Could you check a few things on this model? Use its own coordinates, in mm. A direction names the side the tool comes from. Coordinates: 2 decimals unless noted, no trailing zeros. Write each loop counter-clockwise with the first axis right and the second up, starting at its lowest first coordinate (ties: lowest second). Pieces come first, ordered by that corner, then holes.
Item 1: For P1, Ø3, axis at x = 7, z = 11.5, coming from the +Y side; P2, Ø6.5, axis at y = 8, z = 7.5, coming from the +X side; P3, Ø1, axis at x = 3, z = 10, coming from the +Y side; P4, Ø3, axis at y = -24.5, z = 5.5, coming from the -X side, each with a flat end and sliding along its axis, tell me the tip position at first contact or that it passes through.
Item 2: I want a section at A-A on z = 7.5. Please give me the cut outline in (x, y), then the cut area to 4 significant figures.
Item 3: Thinking about a two-plate mould opening in Z: for faces 4 (the flat face through (10, -13, 15)), 5 (the cylindrical face through (2.46, 6.39, 11.38)), 6 (the flat face through (2.5, 15, 7.5)), which applies, +Z half, -Z half, draft (parallel to the pull), parting line (faces both ways), or undercut?
Item 4: I want a section at B-B on x = 2.25. Please give me the cut outline in (y, z), then the cut area to 3 significant figures.
Item 5: Which directions (+Z, -Z, +X, -X, +Y, -Y) give clear straight access to the entire face, cutting with the end or side of a thin tool? Please do faces 1 (the flat face through (9, 0, 7)), 2 (the flat face through (11, -35, 7)), 3 (the flat face through (4, -5, 7)).
Item 6: I want a section at D-D on x = 10.5. Please give me the cut outline in (y, z).
Item 7: If I drill on probe 1 along Y at (x, z) = (3.15, 7.5); probe 2 along Z at (x, y) = (1.4, 8); probe 3 along X at (y, z) = (-33, 9), over which ranges is the centre line in solid material (lowest first)?
Item 8: I want a section at C-C on y = -20. Please give me the cut outline in (x, z), then the cut area to 3 significant figures.
Solid Edge part; units mm, degrees
sketch "Sketch1" plane through (0, 0, 0) normal (0, -1, 0) x (1, 0, 0)
  line L0 (13.5, 0) -> (0, 0)
  line L1 (0, 0) -> (0, 15)
  line L2 (0, 15) -> (13.5, 15)
  line L3 (13.5, 15) -> (13.5, 0)
extrude "Protrusion1" add sketch "Sketch1" along normal blind 5
sketch "Sketch2" plane through (18.75, -5, 7.5) normal (0, -1, 0) x (1, 0, 0)
  line L0 (-10.25, -7.5) -> (-10.25, 7.5)
  line L1 (-10.25, 7.5) -> (-5.25, 7.5)
  line L2 (-5.25, 7.5) -> (-5.25, -7.5)
  line L3 (-5.25, -7.5) -> (-10.25, -7.5)
extrude "ExtrudedProtrusion_2" add sketch "Sketch2" along normal blind 30
sketch "Sketch3" plane through (18.75, 0, 7.5) normal (0, 1, 0) x (-1, 0, 0)
  line L0 (13.75, -7.5) -> (13.75, 7.5)
  line L1 (13.75, 7.5) -> (18.75, 7.5)
  line L2 (18.75, 7.5) -> (18.75, -7.5)
  line L3 (18.75, -7.5) -> (13.75, -7.5)
extrude "ExtrudedProtrusion_3" add sketch "Sketch3" along normal blind 15
sketch "Sketch4" plane through (13.5, -17.5, 7.5) normal (1, 0, 0) x (0, 1, 0)
  circle A0 centre (-2.5, 0) radius 4
extrude "Cutout1" cut sketch "Sketch4" against normal through all
sketch "Sketch5" plane through (0, 5, 7.5) normal (-1, 0, 0) x (0, -1, 0)
  circle A0 centre (-3, 0) radius 4
extrude "Cutout2" cut sketch "Sketch5" against normal through all
fillet "Round1" radius 7 2 edges at (2.5, 15, 15) (2.5, 15, 0)
hole "Hole_1" at (0, 8, 7.5) direction (1, 0, 0) diameter 8.4 end up to next
hole "Hole_2" at (13.5, -20, 7.5) direction (-1, 0, 0) diameter 8.4 end up to next
Response values:
1. P1: stops at y = 0
1. P2: passes through
1. P3: stops at y = 14.84
1. P4: stops at x = 8.5
2. outline: (0, -5) - (8.5, -5) - (8.5, -15.8) - (13.5, -15.8) - (13.5, 0) - (5, 0) - (5, 3.8) - (0, 3.8) - close; (0, 12.2) - (5, 12.2) - (5, 15) - (0, 15) - close; (8.5, -35) - (13.5, -35) - (13.5, -24.2) - (8.5, -24.2) - close
2. area: 208.5 mm2
3. face 4: +Z half
3. face 5: undercut
3. face 6: draft
4. outline: (-5, 0) - (8, 0) arc R7 ccw to (15, 7) - (15, 8) arc R7 ccw to (8, 15) - (-5, 15) - close; hole circle Ø8.4 at (8, 7.5)
4. area: 224 mm2
5. face 1: +Z, -Z, +X, +Y
5. face 2: +Z, -Z, +X, -X, -Y
5. face 3: +Z, -Z, -X, -Y
6. outline: (-35, 0) - (0, 0) - (0, 15) - (-35, 15) - close; hole circle Ø8.4 at (-20, 7.5)
7. probe 1: y = -5 to 3.8, 12.2 to 15
7. probe 2: z = 0 to 3.3, 11.7 to 15
7. probe 3: x = 8.5 to 13.5
8. outline: (8.5, 0) - (13.5, 0) - (13.5, 3.3) - (8.5, 3.3) - close; (8.5, 11.7) - (13.5, 11.7) - (13.5, 15) - (8.5, 15) - close
8. area: 33.0 mm2
